The listing builds one solid part. Answer for the finished solid, in the listing's coordinates (mm). A direction names the side the tool comes from. Round coordinates to 2 decimals unless told otherwise and drop trailing zeros. Write each loop counter-clockwise with the first axis right and the second up, starting at its lowest first coordinate (ties: lowest second). Pieces come first, ordered by that corner, then holes.
from build123d import *
from build123d.topology import SkipClean

# Parameters (mm, degrees)
BOSS_EXTRUDE2_DEPTH            = 10
SKETCH3_R                      = 40
SKETCH3_R_2                    = 37
BOSS_EXTRUDE3_DEPTH            = 20.040152
CUT_EXTRUDE1_REACH             = 115.803
CUT_EXTRUDE1_END_RADIUS        = 37
SKETCH5_R                      = 1.74703634
SKETCH5_R_2                    = 1.683355043
SKETCH10_W                     = 30.914979244
SKETCH10_H                     = 10
BOSS_EXTRUDE8_DEPTH            = 6
SKETCH11_W                     = 30.914979244
SKETCH11_H                     = 10
BOSS_EXTRUDE9_DEPTH            = 6
SKETCH12_W                     = 10
SKETCH12_H                     = 32.040152213
BOSS_EXTRUDE10_DEPTH           = 6
SKETCH13_W                     = 10
SKETCH13_H                     = 32.040152213
BOSS_EXTRUDE11_DEPTH           = 6
FILLET3_R                      = 6
BOSS_EXTRUDE12_REACH           = 108.364
BOSS_EXTRUDE13_REACH           = 108.364
SKETCH17_R                     = 6.5
CUT_EXTRUDE3_DEPTH             = 5
CUT_EXTRUDE3_DIRECTION_2_REACH = 108.364
CUT_EXTRUDE4_REACH             = 108.364
CUT_EXTRUDE4_END_RADIUS        = 37
FILLET4_R                      = 3
CUT_EXTRUDE5_REACH             = 115.803
FILLET5_R                      = 10


with BuildPart() as part:
    # Sketch1 → Boss-Extrude2 (new body)
    with BuildSketch(Plane.XY):
        Polygon((-3.075119388, 21.362598398), (19.547102475, 0.291978577), (33.205802521, 14.956480402), (10.583580658, 36.027100222), align=None)
    extrude(amount=BOSS_EXTRUDE2_DEPTH)

    # Sketch3 → Boss-Extrude3 (add)
    with BuildSketch(Plane(origin=(22.884598517, 24.569778644, 0), x_dir=(-0.7317560100777086, 0.6815666817818727, 0), z_dir=(0.6815666817818727, 0.7317560100777086, 0))):
        with Locations((1.352782776, 46.892628188)):
            Circle(SKETCH3_R)
        with Locations((1.352782776, 46.892628188)):
            Circle(SKETCH3_R_2, mode=Mode.SUBTRACT)
    extrude(amount=-BOSS_EXTRUDE3_DEPTH)

    # Cut-Extrude1: up to this cylinder (the profile starts outside it)
    cut_extrude1_end = Plane(origin=(15.043707154, 18.136311869, 46.892628188), z_dir=(0.6815666817818727, 0.7317560100777086, 0)) * Cylinder(CUT_EXTRUDE1_END_RADIUS, 323.139339437, mode=Mode.PRIVATE)
    # Sketch5 → Cut-Extrude1 (cut, up to the surface)
    with BuildSketch(Plane(origin=(0, 0, 0), x_dir=(-1, 0, 0), z_dir=(0, 0, -1)), mode=Mode.PRIVATE) as cut_extrude1_sk1:
        with Locations((-13.552748015, 30.82203985)):
            Circle(SKETCH5_R)
    cut_extrude1_tool1 = extrude(cut_extrude1_sk1.sketch, amount=-CUT_EXTRUDE1_REACH, mode=Mode.PRIVATE) - cut_extrude1_end
    add(cut_extrude1_tool1.solids().sort_by_distance((13.552748, 30.82204, 0))[0], mode=Mode.SUBTRACT)
    # Sketch5 → Cut-Extrude1 (cut, up to the surface)
    with BuildSketch(Plane(origin=(0, 0, 0), x_dir=(-1, 0, 0), z_dir=(0, 0, -1)), mode=Mode.PRIVATE) as cut_extrude1_sk2:
        with Locations((-2.306822594, 18.748043967)):
            Circle(SKETCH5_R)
    cut_extrude1_tool2 = extrude(cut_extrude1_sk2.sketch, amount=-CUT_EXTRUDE1_REACH, mode=Mode.PRIVATE) - cut_extrude1_end
    add(cut_extrude1_tool2.solids().sort_by_distance((2.306823, 18.748044, 0))[0], mode=Mode.SUBTRACT)
    # Sketch5 → Cut-Extrude1 (cut, up to the surface)
    with BuildSketch(Plane(origin=(0, 0, 0), x_dir=(-1, 0, 0), z_dir=(0, 0, -1)), mode=Mode.PRIVATE) as cut_extrude1_sk3:
        with Locations((-17.810962495, 4.261826269)):
            Circle(SKETCH5_R_2)
    cut_extrude1_tool3 = extrude(cut_extrude1_sk3.sketch, amount=-CUT_EXTRUDE1_REACH, mode=Mode.PRIVATE) - cut_extrude1_end
    add(cut_extrude1_tool3.solids().sort_by_distance((17.810962, 4.261826, 0))[0], mode=Mode.SUBTRACT)
    # Sketch5 → Cut-Extrude1 (cut, up to the surface)
    with BuildSketch(Plane(origin=(0, 0, 0), x_dir=(-1, 0, 0), z_dir=(0, 0, -1)), mode=Mode.PRIVATE) as cut_extrude1_sk4:
        with Locations((-29.017899523, 16.394033311)):
            Circle(SKETCH5_R)
    cut_extrude1_tool4 = extrude(cut_extrude1_sk4.sketch, amount=-CUT_EXTRUDE1_REACH, mode=Mode.PRIVATE) - cut_extrude1_end
    add(cut_extrude1_tool4.solids().sort_by_distance((29.0179, 16.394033, 0))[0], mode=Mode.SUBTRACT)

    # Sketch10 → Boss-Extrude8 (add)
    with BuildSketch(Plane(origin=(9.22589847, 9.905276819, 0), x_dir=(0.7317560100777085, -0.6815666817818729, 0), z_dir=(-0.6815666817818729, -0.7317560100777085, 0))):
        with Locations((-1.352782776, 5)):
            Rectangle(SKETCH10_W, SKETCH10_H)
    extrude(amount=BOSS_EXTRUDE8_DEPTH)

    # Sketch11 → Boss-Extrude9 (add)
    with BuildSketch(Plane(origin=(22.884598517, 24.569778644, 0), x_dir=(0.7317560100777083, -0.681566681781873, 0), z_dir=(0.681566681781873, 0.7317560100777083, 0))):
        with Locations((-1.352782776, -5)):
            Rectangle(SKETCH11_W, SKETCH11_H)
    extrude(amount=BOSS_EXTRUDE9_DEPTH)

    # Sketch12 → Boss-Extrude10 (add)
    with BuildSketch(Plane(origin=(-12.301017858, 11.457321578, 0), x_dir=(0, 0, 1), z_dir=(-0.7317560100777086, 0.6815666817818726, 0))):
        with Locations((5, 23.556386958)):
            Rectangle(SKETCH12_W, SKETCH12_H)
    extrude(amount=BOSS_EXTRUDE10_DEPTH)

    # Sketch13 → Boss-Extrude11 (add)
    with BuildSketch(Plane(origin=(10.321204005, -9.613298242, 0), x_dir=(0, 0, -1), z_dir=(0.7317560100777092, -0.6815666817818721, 0))):
        with Locations((-5, 23.556386958)):
            Rectangle(SKETCH13_W, SKETCH13_H)
    extrude(amount=BOSS_EXTRUDE11_DEPTH)

    # Fillet3
    fillet3_edges = [part.edges().sort_by_distance(p)[0] for p in [
        (10.282444688, 44.507036374, 5),
        (-11.555055539, 21.061462428, 5),
        (41.685738672, 15.257616372, 5),
        (19.848238445, -8.187957574, 5),
    ]]
    fillet(fillet3_edges, radius=FILLET3_R)

    # Sketch15 → Boss-Extrude12 (add, up to next)
    with BuildSketch(Plane.XY.offset(10), mode=Mode.PRIVATE) as boss_extrude12_sk1:
        Polygon((19.547102475, 0.291978577), (23.937638536, -3.797421514), (37.596338582, 10.867080311), (33.205802521, 14.956480402), align=None)
    boss_extrude12_tool1 = extrude(boss_extrude12_sk1.sketch, amount=BOSS_EXTRUDE12_REACH, mode=Mode.PRIVATE) - part.part
    add(boss_extrude12_tool1.solids().sort_by_distance((28.571721, 5.579529, 10))[0])

    # Sketch16 → Boss-Extrude13 (add, up to next)
    with BuildSketch(Plane.XY.offset(10), mode=Mode.PRIVATE) as boss_extrude13_sk1:
        Polygon((10.583580658, 36.027100222), (6.193044598, 40.116500313), (-7.465655449, 25.451998488), (-3.075119388, 21.362598398), align=None)
    boss_extrude13_tool1 = extrude(boss_extrude13_sk1.sketch, amount=BOSS_EXTRUDE13_REACH, mode=Mode.PRIVATE) - part.part
    add(boss_extrude13_tool1.solids().sort_by_distance((1.558963, 30.739549, 10))[0])

    # Sketch17 → Cut-Extrude3 (cut)
    with BuildSketch(Plane.XY.offset(10)):
        with Locations(Location((2.306822594, 18.748043967, 0), (0, 0, 152.697494073))):
            Circle(SKETCH17_R)
        with Locations(Location((13.552748015, 30.82203985, 0), (0, 0, 121.093351503))):
            Circle(SKETCH17_R)
        with Locations(Location((17.810962495, 4.261826269, 0), (0, 0, 152.393126662))):
            Circle(SKETCH17_R)
        with Locations(Location((29.017899523, 16.394033311, 0), (0, 0, 120.935167822))):
            Circle(SKETCH17_R)
    extrude(amount=-CUT_EXTRUDE3_DEPTH, mode=Mode.SUBTRACT)

    # Sketch17 → Cut-Extrude3 direction 2 (cut, up to next)
    with BuildSketch(Plane.XY.offset(10), mode=Mode.PRIVATE) as cut_extrude3_direction_2_sk1:
        with Locations(Location((2.306822594, 18.748043967, 0), (0, 0, 152.697494073))):
            Circle(SKETCH17_R)
    cut_extrude3_direction_2_tool1 = extrude(cut_extrude3_direction_2_sk1.sketch, amount=CUT_EXTRUDE3_DIRECTION_2_REACH, mode=Mode.PRIVATE) & part.part
    # Sketch17 → Cut-Extrude3 direction 2 (cut, up to next)
    with BuildSketch(Plane.XY.offset(10), mode=Mode.PRIVATE) as cut_extrude3_direction_2_sk2:
        with Locations(Location((13.552748015, 30.82203985, 0), (0, 0, 121.093351503))):
            Circle(SKETCH17_R)
    cut_extrude3_direction_2_tool2 = extrude(cut_extrude3_direction_2_sk2.sketch, amount=CUT_EXTRUDE3_DIRECTION_2_REACH, mode=Mode.PRIVATE) & part.part
    # Sketch17 → Cut-Extrude3 direction 2 (cut, up to next)
    with BuildSketch(Plane.XY.offset(10), mode=Mode.PRIVATE) as cut_extrude3_direction_2_sk3:
        with Locations(Location((17.810962495, 4.261826269, 0), (0, 0, 152.393126662))):
            Circle(SKETCH17_R)
    cut_extrude3_direction_2_tool3 = extrude(cut_extrude3_direction_2_sk3.sketch, amount=CUT_EXTRUDE3_DIRECTION_2_REACH, mode=Mode.PRIVATE) & part.part
    # Sketch17 → Cut-Extrude3 direction 2 (cut, up to next)
    with BuildSketch(Plane.XY.offset(10), mode=Mode.PRIVATE) as cut_extrude3_direction_2_sk4:
        with Locations(Location((29.017899523, 16.394033311, 0), (0, 0, 120.935167822))):
            Circle(SKETCH17_R)
    cut_extrude3_direction_2_tool4 = extrude(cut_extrude3_direction_2_sk4.sketch, amount=CUT_EXTRUDE3_DIRECTION_2_REACH, mode=Mode.PRIVATE) & part.part
    add(cut_extrude3_direction_2_tool1.solids().sort_by_distance((2.306823, 18.748044, 10))[0], mode=Mode.SUBTRACT)
    add(cut_extrude3_direction_2_tool2.solids().sort_by_distance((13.552748, 30.82204, 10))[0], mode=Mode.SUBTRACT)
    add(cut_extrude3_direction_2_tool3.solids().sort_by_distance((17.810962, 4.261826, 10))[0], mode=Mode.SUBTRACT)
    add(cut_extrude3_direction_2_tool4.solids().sort_by_distance((29.0179, 16.394033, 10))[0], mode=Mode.SUBTRACT)

    # Cut-Extrude4: up to this cylinder (the profile starts outside it)
    with SkipClean():  # the faces are left unmerged after this step: merging them gives an invalid solid
        cut_extrude4_end = Plane(origin=(15.133329832, 18.232534198, 46.892628188), z_dir=(0.6815666817818727, 0.7317560100777086, 0)) * Cylinder(CUT_EXTRUDE4_END_RADIUS, 291.728, mode=Mode.PRIVATE)
        # Sketch18 → Cut-Extrude4 (cut, up to the surface)
        with BuildSketch(Plane.XY.offset(10), mode=Mode.PRIVATE) as cut_extrude4_sk1:
            Polygon((21.393947235, -1.428195685), (-3.645697664, 21.894042126), (10.148979711, 36.704534402), (35.18862461, 13.382296591), align=None)
        cut_extrude4_tool1 = extrude(cut_extrude4_sk1.sketch, amount=CUT_EXTRUDE4_REACH, mode=Mode.PRIVATE) - cut_extrude4_end
        add(cut_extrude4_tool1.solids().sort_by_distance((15.771463, 17.638169, 10))[0], mode=Mode.SUBTRACT)
        add(cut_extrude4_tool1.solids().sort_by_distance((15.771463, 17.638169, 10))[1], mode=Mode.SUBTRACT)
    add(part.part.scale(1), mode=Mode.REPLACE)  # the faces are merged on a copy

    # Fillet4
    fillet4_edges = [part.edges().sort_by_distance(p)[0] for p in [
        (30.766988562, 3.534829402, 13.135019577),
        (-0.636305422, 32.784249404, 13.135019577),
        (3.18365236, 29.226293038, 13.645787353),
        (28.223297258, 5.904055227, 14.555786818),
    ]]
    fillet(fillet4_edges, radius=FILLET4_R)

    # Sketch19 → Cut-Extrude5 (cut, up to next)
    with BuildSketch(Plane(origin=(0, 0, 0), x_dir=(-1, 0, 0), z_dir=(0, 0, -1)), mode=Mode.PRIVATE) as cut_extrude5_sk1:
        with BuildLine():
            Line((-31.678269443, 24.578698129), (-21.538760737, 34.022763101))
            ThreePointArc((-21.538760737, 34.022763101), (-25.245381726, 27.837218595), (-31.678269443, 24.578698129))
        make_face()
    cut_extrude5_tool1 = extrude(cut_extrude5_sk1.sketch, amount=-CUT_EXTRUDE5_REACH, mode=Mode.PRIVATE) & part.part
    # Sketch19 → Cut-Extrude5 (cut, up to next)
    with BuildSketch(Plane(origin=(0, 0, 0), x_dir=(-1, 0, 0), z_dir=(0, 0, -1)), mode=Mode.PRIVATE) as cut_extrude5_sk2:
        with BuildLine():
            Line((0.30653048, 10.58444578), (-9.832978226, 1.140380807))
            ThreePointArc((-9.832978226, 1.140380807), (-6.126357236, 7.325925314), (0.30653048, 10.58444578))
        make_face()
    cut_extrude5_tool2 = extrude(cut_extrude5_sk2.sketch, amount=-CUT_EXTRUDE5_REACH, mode=Mode.PRIVATE) & part.part
    add(cut_extrude5_tool1.solids().sort_by_distance((26.059499, 28.711286, 0))[0], mode=Mode.SUBTRACT)
    add(cut_extrude5_tool2.solids().sort_by_distance((5.31224, 6.451858, 0))[0], mode=Mode.SUBTRACT)

    # Fillet5
    fillet5_edges = [part.edges().sort_by_distance(p)[0] for p in [
        (21.538760737, 34.022763101, 5),
        (31.678269443, 24.578698129, 5),
        (9.832978226, 1.140380807, 5),
        (-0.30653048, 10.58444578, 5),
    ]]
    fillet(fillet5_edges, radius=FILLET5_R)


solid = part.part
1. Section B-B on z = 54 is taken. Determine the outline of the cut face in (x, y), plus the area to 3 significant figures.
Geometry says:
outline: (-20.57, 37.66) - (-18.33, 35.58) - (-4.68, 50.24) - (-6.91, 52.32) - close; (34.81, -13.92) - (37.04, -16) - (50.7, -1.34) - (48.47, 0.74) - close
area: 122 mm2
2. A tool of negligible diameter and unlimited length cuts with its end or side. For faces 4 (the face through (28.32, 6.01, 11.4)), 5 (the face through (29.5, 18.3, 5)), 6 (the face through (13.931, 29.117, 2.465)), from which of +Z, -Z, +X, -X, +Y, -Y can it reach the whole face along a straight path? Write none if from no direction.
Geometry says:
face 4: -X, +Y
face 5: none
face 6: -Z
3. Straight lines are drawn through the part: line 1 along Z through (x, y) = (-2.5, 31); line 2 along Z through (x, y) = (12, 35.5); line 3 along Z through (x, y) = (2, 35.5). For each, find the intervals that lie inside material, in ascending order.
Geometry says:
line 1: z = 12.46 to 16.86, 76.93 to 80.56
line 2: z = 0 to 5
line 3: z = 0 to 16.69, 77.09 to 80.7
4. Given pin 1 (3 mm diameter, centred on x = 32.5, z = 31, fed in from +Y); pin 2 (14.5 mm diameter, centred on x = 29, y = 13.5, fed in from +Z); pin 3 (6 mm diameter, centred on x = 39.5, z = 26.5, fed in from +Y), each flat-ended and moving along its own axis, determine where each tip first touches the part or whether it passes through.
Geometry says:
pin 1: stops at y = -10.21
pin 2: stops at z = 86.42
pin 3: stops at y = 3.59
5. For a pull along Y with two mould halves and no side action, classify faces 1 (the face through (-0.4, 10.98, 5.07)), 2 (the face through (17.17, 38.09, 5.07)), 3 (the face through (22.52, 16.57, 7.54)) as released by +Y, released by -Y, zero draft, split by the parting line, or undercut.
Geometry says:
face 1: released by -Y
face 2: released by +Y
face 3: undercut
6. Section A-A on z = 17 is taken. Determine the outline of the cut face in (x, y), plus the area to 3 significant figures.
Geometry says:
outline: (-11.21, 28.94) - (-7.72, 25.69) - (5.94, 40.35) - (2.45, 43.61) - close; (24.19, -4.03) - (27.69, -7.29) - (41.34, 7.38) - (37.85, 10.63) - close
area: 191 mm2
